Check sheet for the modelled part. Datum: model origin and axes. Units: mm. Coordinates: 2 decimals unless noted, no trailing zeros. Write each loop counter-clockwise with the first axis right and the second up, starting at its lowest first coordinate (ties: lowest second). Pieces come first, ordered by that corner, then holes. Notation, with made-up numbers: M -18.75,79 L 6.25,79 A17 cw 6.25,97 Z; hole C -13.75,-2.5 d10. An arc over 180 degrees is marked long. Answer as CSV lines item,"result". Start each with the question number.
Q1. Depth check by flat-ended pin: pin 1 Ø1.5 at (x, y) = (14.5, 415) entering from -Z; pin 2 Ø1.5 at (x, y) = (40, 38) entering from -Z. Enter the tip coordinate at first touch or a pass-through.
Q2. Sectioned sample at C-C, the plane z = 2.15. Count the separate pieces of the cut face and the enclosed holes in it, then the cut area to 3 significant figures.
Q3. Thickness scan on line 1 along X through (y, z) = (22, 3.05); line 2 along X through (y, z) = (250, 2); line 3 along X through (y, z) = (205.5, 0.85). Record the ranges inside material, lowest first. Write a range as from..to.
Q4. Sectioned sample at A-A, the plane x = 24.25. Record the cut outline in (y, z).
Q5. Sectioned sample at B-B, the plane y = 180.5. Record the cut outline in (x, z).
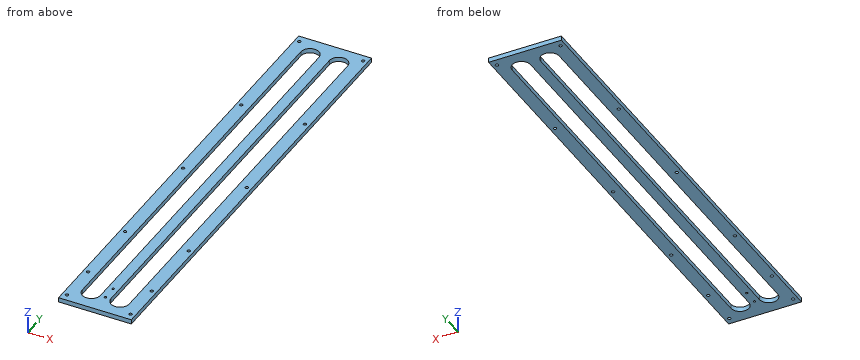
Autodesk Inventor part; units mm, degrees
ref_plane "YZ Plane" through (0, 0, 0) normal (1, 0, 0) x (0, 1, 0)
ref_plane "XZ Plane" through (0, 0, 0) normal (0, 1, 0) x (-1, 0, 0)
ref_plane "XY Plane" through (0, 0, 0) normal (0, 0, 1) x (1, 0, 0)
sketch "Sketch1" plane through (0, 0, 0) normal (0, 0, 1) x (1, 0, 0)
  line L0 (0, 0) -> (80, 0)
  line L1 (80, 0) -> (80, 500)
  line L2 (80, 500) -> (0, 500)
  line L3 (0, 500) -> (0, 0)
  line L4 (40, 500) -> (40, 0) construction
  line L5 (24.25, 477.5) -> (24.25, 22.5) construction
  line L6 (14.25, 477.5) -> (14.25, 22.5)
  line L7 (34.25, 22.5) -> (34.25, 477.5)
  arc A0 (34.25, 477.5) -> (14.25, 477.5) centre (24.25, 477.5) ccw
  arc A1 (14.25, 22.5) -> (34.25, 22.5) centre (24.25, 22.5) ccw
  circle A2 centre (5, 52) radius 2.5 construction
  circle A3 centre (5, 8) radius 2.5 construction
  line L8 (65.75, 477.5) -> (65.75, 22.5)
  line L9 (45.75, 22.5) -> (45.75, 477.5)
  arc A4 (65.75, 477.5) -> (45.75, 477.5) centre (55.75, 477.5) ccw
  arc A5 (45.75, 22.5) -> (65.75, 22.5) centre (55.75, 22.5) ccw
  circle A6 centre (75, 52) radius 2.5 construction
  circle A7 centre (75, 8) radius 2.5 construction
  circle A8 centre (5, 492) radius 1 construction
  circle A9 centre (75, 492) radius 1 construction
  line L10 (5, 8) -> (5, 52) construction
  circle A10 centre (5, 371) radius 1 construction
  circle A11 centre (75, 371) radius 1 construction
  circle A12 centre (5, 250) radius 1 construction
  circle A13 centre (75, 250) radius 1 construction
  circle A14 centre (5, 129) radius 1 construction
  circle A15 centre (75, 129) radius 1 construction
  circle A16 centre (5, 8) radius 1 construction
  circle A17 centre (75, 8) radius 1 construction
  line L11 (75, 8) -> (75, 52) construction
  line L12 (0, 500) -> (10, 500) construction
  line L13 (10, 500) -> (10, 0) construction
  line L14 (10, 0) -> (0, 0) construction
  line L15 (0, 0) -> (0, 500) construction
  line L16 (80, 500) -> (70, 500) construction
  line L17 (70, 500) -> (70, 0) construction
  line L18 (70, 0) -> (80, 0) construction
  line L19 (80, 0) -> (80, 500) construction
  line L20 (5, 8) -> (75, 8) construction
  line L21 (5, 8) -> (75, 8) construction
  point P0 (24.25, 250)
  dimension "d0" = 500
  dimension "d1" = 80
  dimension "d2" = 10
  dimension "d6" = 5
  dimension "d7" = 5
  dimension "d10" = 44
  dimension "d12" = 31.5
  dimension "d17" = 2
  dimension "d18" = 5
  dimension "d19" = 8
  dimension "d27" = 455
  dimension "d28" = 250
  dimension "d32" = 121
  dimension "d45" = 10
  dimension "d46" = 10
  dimension "d54" = 70
extrude "Extrusion1" add sketch "Sketch1" along normal blind 5
hole "Bohrung1" at (5, 52, 0) at (5, 8, 0) at (75, 8, 0) at (75, 52, 0) direction (0, 0, 1) diameter 3.4 depth 11.8 tip angle 118
hole "Bohrung2" at (5, 492, 0) at (75, 492, 0) at (5, 371, 0) at (75, 371, 0) at (5, 250, 0) at (75, 250, 0) at (5, 129, 0) at (75, 129, 0) at (5, 8, 0) at (75, 8, 0) direction (0, 0, 1) diameter 3.4 end through all
ref_plane "Arbeitsebene2" through (5, 30, 5.9) normal (0, 1, 0) x (0, 0, 1)
ref_plane "Arbeitsebene1" through (5, 8, 5.9) normal (0, 1, 0) x (0, 0, 1)
sketch "Skizze2" plane through (0, 0, 5) normal (0, 0, 1) x (1, 0, 0)
  line L0 (-16, 30) -> (96, 30) construction
  line L1 (40, 500) -> (40, 0) construction
  point P0 (0, 0)
  point P1 (40, 38)
  point P2 (40, 22)
  dimension "d56" = 8
  dimension "d57" = 8
hole "Bohrung3" at (40, 22, 5) at (40, 38, 5) direction (0, 0, -1) diameter 2.459 depth 8.8 tip angle 118
equation "\"d0\" = GuidanceTrack_Length"
equation "\"d1\" = BackPlate_Width"
equation "\"d18\" = 0.5 * GuidanceTrac_OneSide_Thickness"
equation "\"d19\" = TopLit_Fixhole_Edge_Dist"
equation "\"d54\" = Guidacne_fixHoleDist"
properties part number "Slot profile" material "PMMA-Kunststoff"
Output:
1,pin 1,"stops at z = 0"
1,pin 2,"passes through"
2,separate pieces,"1"
2,enclosed holes,"16"
2,area,"21,100 mm^2"
3,line 1,"x = 0..14.26, 34.24..38.77, 41.23..45.76, 65.74..80"
3,line 2,"x = 0..3.3, 6.7..14.25, 34.25..45.75, 65.75..73.3, 76.7..80"
3,line 3,"x = 0..14.25, 34.25..45.75, 65.75..80"
4,outline,"M 0,0 L 12.5,0 L 12.5,5 L 0,5 Z; M 487.5,0 L 500,0 L 500,5 L 487.5,5 Z"
5,outline,"M 0,0 L 14.25,0 L 14.25,5 L 0,5 Z; M 34.25,0 L 45.75,0 L 45.75,5 L 34.25,5 Z; M 65.75,0 L 80,0 L 80,5 L 65.75,5 Z"
